For this review, take the finished solid that the model builds, in its own axes (mm). Coordinates: 2 decimals unless noted, no trailing zeros. Loops run counter-clockwise (first coordinate to the right, second up) from the corner with the lowest first, then second, coordinate; pieces in that order, holes last. Notation, with made-up numbers: (5.5, 34) -> (11.5, 34) arc R13 cw to (11.5, 41) -> close; hole circle Ø1 at (75.5, 84). An arc over 180 degrees is marked (long way). One line per item, written item: value.
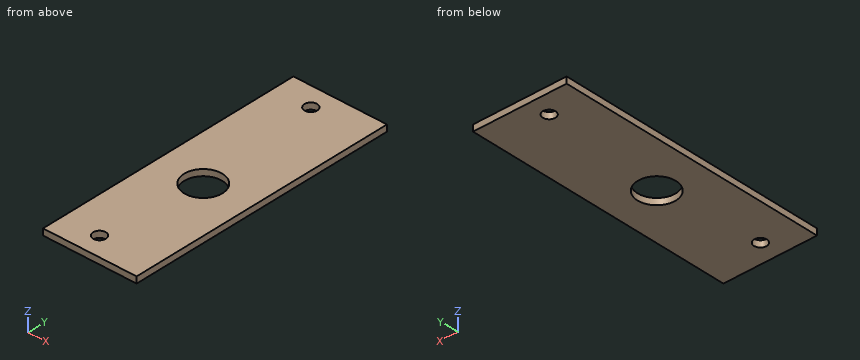
Autodesk Inventor part; units mm, degrees
ref_plane "YZ Plane" through (0, 0, 0) normal (1, 0, 0) x (0, 1, 0)
ref_plane "XZ Plane" through (0, 0, 0) normal (0, 1, 0) x (-1, 0, 0)
ref_plane "XY Plane" through (0, 0, 0) normal (0, 0, 1) x (1, 0, 0)
sketch "スケッチ1" plane through (0, 0, 0) normal (0, 0, 1) x (1, 0, 0)
  line L0 (11, -32) -> (-11, -32)
  line L1 (-11, -32) -> (-11, 32)
  line L2 (-11, 32) -> (11, 32)
  line L3 (11, 32) -> (11, -32)
  line L4 (11, -32) -> (-11, 32) construction
  line L5 (-11, -32) -> (11, 32) construction
  point P0 (0, 0)
  dimension "d0" = 22
  dimension "d1" = 64
extrude "押し出し1" add sketch "スケッチ1" along normal blind 1.5
sketch "スケッチ2" plane through (0, 0, 1.5) normal (0, 0, 1) x (1, 0, 0)
  line L0 (-11, 32) -> (-11, -32)
  line L1 (11, 32) -> (-11, 32)
  line L2 (-11, -32) -> (11, -32)
  point P0 (0, 0)
  point P1 (-2.3, 27)
  point P2 (-2.3, -27)
  dimension "d4" = 8.7
  dimension "d5" = 5
  dimension "d6" = 5
hole "穴1" at (-2.3, 27, 1.5) at (-2.3, -27, 1.5) direction (0, 0, -1) diameter 3 end through all
sketch "スケッチ3" plane through (0, 0, 1.5) normal (0, 0, 1) x (1, 0, 0)
  circle A0 centre (0, -3) radius 4.5
  line L0 (11, 32) -> (-11, 32)
  point P0 (0, 0)
  dimension "d14" = 35
  dimension "d15" = 9
extrude "押し出し2" cut sketch "スケッチ3" against normal blind 1.5
properties part number "pcb_base" material "アルミニウム 6061"
1. Take a section at C-C, the plane y = -3. Give the boundary of the cut face in (x, z).
Return value:
outline: (-11, 0) -> (-4.5, 0) -> (-4.5, 1.5) -> (-11, 1.5) -> close; (4.5, 0) -> (11, 0) -> (11, 1.5) -> (4.5, 1.5) -> close
2. Take a section at A-A, the plane x = 0. Give the boundary of the cut face in (y, z), and give its area (3 significant figures).
Return value:
outline: (-32, 0) -> (-7.5, 0) -> (-7.5, 1.5) -> (-32, 1.5) -> close; (1.5, 0) -> (32, 0) -> (32, 1.5) -> (1.5, 1.5) -> close
area: 82.5 mm2
3. Insertion check: pin 1 Ø2.5 at (x, y) = (-2.3, 27) entering from +Z. The pin has a flat end and moves straight along its axis. Give the tip position at first contact, or say it passes through.
Return value:
pin 1: passes through
4. To check wall thickness, follow probe 1 along X at (y, z) = (-27, 0.9); probe 2 along Y at (x, z) = (-2.3, 0.9); probe 3 along Y at (x, z) = (-3, 0.95). State the ranges of each line that lie inside material, in increasing order. Write a range as from..to.
Return value:
probe 1: x = -11..-3.8, -0.8..11
probe 2: y = -32..-28.5, -25.5..-6.87, 0.87..25.5, 28.5..32
probe 3: y = -32..-28.33, -25.67..-6.35, 0.35..25.67, 28.33..32
5. Take a section at B-B, the plane z = 1. Give the boundary of the cut face in (x, y), and give its area (3 significant figures).
Return value:
outline: (-11, -32) -> (11, -32) -> (11, 32) -> (-11, 32) -> close; hole circle Ø9 at (0, -3); hole circle Ø3 at (-2.3, -27); hole circle Ø3 at (-2.3, 27)
area: 1,330 mm2
